Geometry check sheet. Reference: drawing and pictorial views, mm from the part's lowest x, y, z. Round coordinates to 2 decimals unless told otherwise and drop trailing zeros. Write each loop counter-clockwise with the first axis right and the second up, starting at its lowest first coordinate (ties: lowest second). Pieces come first, ordered by that corner, then holes. Notation, with made-up numbers: M 38,-9 L 84,-9 A18 cw 84,18 Z; hole C 20,-6 d8. An arc over 180 degrees is marked long. Put each result on its own line as item: value. Start each with the question number.
(1) Section check A-A on z = 16.5. Record the cut outline in (x, y).
(2) Material ranges on probe 1 along X at (y, z) = (0.3, 16.5); probe 2 along X at (y, z) = (0.15, 23); probe 3 along X at (y, z) = (0.15, 8), recorded low to high.
(3) Section check C-C on x = 16.5. Record the cut outline in (y, z).
(4) Section check D-D on z = 23. Record the cut outline in (x, y).
(5) Section check B-B on y = 0.3. Record the cut outline in (x, z).
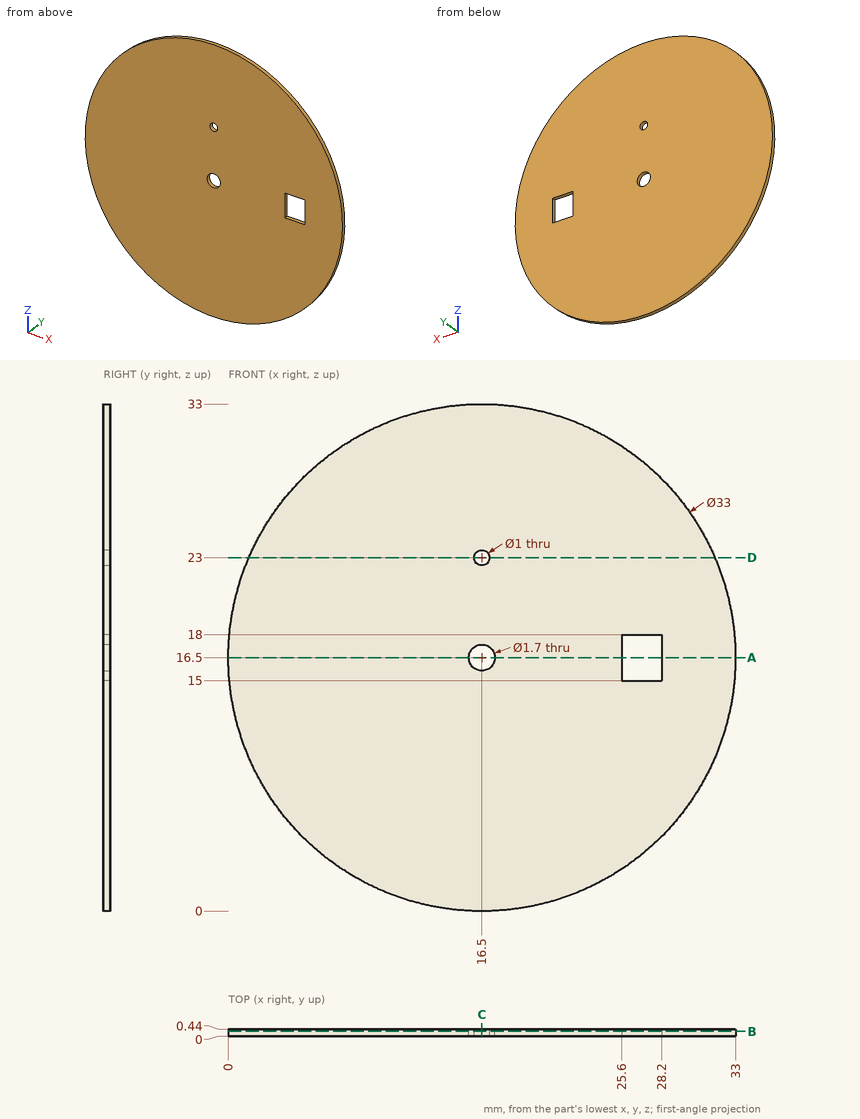
Answers follow:
1. outline: M 0,0 L 15.65,0 L 15.65,0.44 L 0,0.44 Z; M 17.35,0 L 25.6,0 L 25.6,0.44 L 17.35,0.44 Z; M 28.2,0 L 33,0 L 33,0.44 L 28.2,0.44 Z
2. probe 1: x = 0 to 15.65, 17.35 to 25.6, 28.2 to 33
2. probe 2: x = 1.33 to 16, 17 to 31.67
2. probe 3: x = 2.36 to 30.64
3. outline: M 0,0 L 0.44,0 L 0.44,15.65 L 0,15.65 Z; M 0,17.35 L 0.44,17.35 L 0.44,22.5 L 0,22.5 Z; M 0,23.5 L 0.44,23.5 L 0.44,33 L 0,33 Z
4. outline: M 1.33,0 L 16,0 L 16,0.44 L 1.33,0.44 Z; M 17,0 L 31.67,0 L 31.67,0.44 L 17,0.44 Z
5. outline: C 16.5,16.5 d33; hole C 16.5,16.5 d1.7; hole C 16.5,23 d1; hole M 25.6,15 L 28.2,15 L 28.2,18 L 25.6,18 Z
